```python
from build123d import *

# Parameters (mm, degrees)
SKETCH_1_W               = 29
SKETCH_1_H               = 32.7
EXTRUDE_1_DEPTH          = 29
SKETCH_2_R               = 14.5
SKETCH_2_R_2             = 12.5
EXTRUDE_2_DEPTH          = 7
SKETCH_3_R               = 1.5
CUT_EXTRUDE_1_DEPTH      = 5
CUT_EXTRUDE_START        = -2.9
SKETCH_4_R               = 1.5
CUT_EXTRUDE_2_DEPTH      = 2.9
SKETCH_5_R               = 4.3
SKETCH_5_R_2             = 3.5
EXTRUDE_3_DEPTH          = 6.9
SKETCH_6_W               = 16.3
SKETCH_6_H               = 15.8
EXTRUDE_4_DEPTH          = 2
PATTERN_CIRCULAR_1_COUNT = 4


with BuildPart() as part:
    # 草图1 → 凸台-拉伸1 (new body)
    with BuildSketch(Plane(origin=(0, 0, 0), x_dir=(1, 0, 0), z_dir=(0, 1, 0))):
        Rectangle(SKETCH_1_W, SKETCH_1_H)
    extrude(amount=EXTRUDE_1_DEPTH)

    # 草图2 → 凸台-拉伸2 (add)
    with BuildSketch(Plane.XY.offset(16.35)):
        with Locations((0, 14.5)):
            Circle(SKETCH_2_R)
        with Locations((0, 14.5)):
            Circle(SKETCH_2_R_2, mode=Mode.SUBTRACT)
    extrude(amount=EXTRUDE_2_DEPTH)

    # 草图3 → 切除-拉伸1 (cut)
    with BuildSketch(Plane.XZ):
        with Locations(Location((-10, 14.35, 0), (0, 0, 270))):
            Circle(SKETCH_3_R)
        with Locations(Location((10, 14.35, 0), (0, 0, 270))):
            Circle(SKETCH_3_R)
        with Locations(Location((-10, -14.35, 0), (0, 0, 270))):
            Circle(SKETCH_3_R)
        with Locations(Location((10, -14.35, 0), (0, 0, 270))):
            Circle(SKETCH_3_R)
    extrude(amount=-CUT_EXTRUDE_1_DEPTH, mode=Mode.SUBTRACT)

    # 草图4 → 切除-拉伸2 (cut)
    with BuildSketch(Plane(origin=(0, 29, 0), x_dir=(1, 0, 0), z_dir=(0, 1, 0)).offset(CUT_EXTRUDE_START)):
        with Locations(Location((0, 14.35, 0), (0, 0, 270))):
            Circle(SKETCH_4_R)
        with Locations(Location((-10, -14.35, 0), (0, 0, 90))):
            Circle(SKETCH_4_R)
        with Locations(Location((10, -14.35, 0), (0, 0, 90))):
            Circle(SKETCH_4_R)
    cut_extrude_2 = extrude(amount=CUT_EXTRUDE_2_DEPTH, mode=Mode.SUBTRACT)

    # 草图5 → 凸台-拉伸3 (add)
    with BuildSketch(Plane(origin=(0, 0, -16.35), x_dir=(-1, 0, 0), z_dir=(0, 0, -1))):
        with Locations(Location((-7.3, 21.8, 0), (0, 0, 180))):
            Circle(SKETCH_5_R)
        with Locations(Location((-7.3, 21.8, 0), (0, 0, 180))):
            Circle(SKETCH_5_R_2, mode=Mode.SUBTRACT)
    extrude(amount=EXTRUDE_3_DEPTH)

    # 草图6 → 凸台-拉伸4 (add)
    with BuildSketch(Plane(origin=(0, 0, -16.35), x_dir=(-1, 0, 0), z_dir=(0, 0, -1))):
        with Locations((0, 7.9)):
            Rectangle(SKETCH_6_W, SKETCH_6_H)
    extrude(amount=EXTRUDE_4_DEPTH)

    # 阵列(圆周)1: 切除-拉伸2 ×4 about axis, 1 skipped
    pattern_circular_1_axis = Axis((0, 14.5, 0), (0, 0, -1))
    add([cut_extrude_2.rotate(pattern_circular_1_axis, i * 360 / PATTERN_CIRCULAR_1_COUNT) for i in range(1, PATTERN_CIRCULAR_1_COUNT) if i not in (2,)], mode=Mode.SUBTRACT)


solid = part.part
```
Source: CAD feature listing. Evaluate the final solid. Frame: model axes, mm. A direction names the side the tool comes from. Round coordinates to 2 decimals unless told otherwise and drop trailing zeros. Loops run counter-clockwise (first coordinate to the right, second up) from the corner with the lowest first, then second, coordinate; pieces in that order, holes last. Notation, with made-up numbers: (-7.75, -36.75) - (17.25, -36.75) arc R20 cw to (17.25, -21.75) - close; hole circle Ø6 at (11, -24.5). An arc over 180 degrees is marked (long way). Use CSV: the item, a comma, the result in double quotes.
Q1. Section query D-D, the plane x = -3. Output: boundary loops of the cut face in (y, z).
Reported:
outline,"(0, -18.35) - (15.8, -18.35) - (15.8, -16.35) - (29, -16.35) - (29, 16.35) - (28.69, 16.35) - (28.69, 23.35) - (26.63, 23.35) - (26.63, 16.35) - (2.37, 16.35) - (2.37, 23.35) - (0.31, 23.35) - (0.31, 16.35) - (0, 16.35) - close"
Q2. Section query C-C, the plane z = -14.35. Output: boundary loops of the cut face in (x, y).
Reported:
outline,"(-14.5, 0) - (-11.5, 0) - (-11.5, 5) - (-8.5, 5) - (-8.5, 0) - (8.5, 0) - (8.5, 5) - (11.5, 5) - (11.5, 0) - (14.5, 0) - (14.5, 13) - (11.6, 13) - (11.6, 16) - (14.5, 16) - (14.5, 29) - (1.5, 29) - (1.5, 26.1) - (-1.5, 26.1) - (-1.5, 29) - (-14.5, 29) - (-14.5, 16) - (-11.6, 16) - (-11.6, 13) - (-14.5, 13) - close"
Q3. Section query B-B, the plane z = 20. Output: boundary loops of the cut face in (x, y).
Reported:
outline,"circle Ø29 at (0, 14.5); hole circle Ø25 at (0, 14.5)"
Q4. Pin query (flat end, axial travel): pin 1 Ø2 at (x, y) = (-4.5, 23.5) entering from -Z; pin 2 Ø6 at (x, y) = (1.5, 8) entering from -Z; pin 3 Ø7.5 at (x, y) = (6, 18) entering from +Z. Return the tip coordinate at first contact, or that it passes through.
Reported:
pin 1,"z = -16.35"
pin 2,"z = -18.35"
pin 3,"z = 16.35"
Q5. Reachability of faces 4 (the cylindrical face through (-10.07, 27.53, 15.85)), 5 (the cylindrical face through (13.03, 4.57, 15.85)), 6 (the cylindrical face through (-10.91, 2.46, -13.16)), 7 (the cylindrical face through (-13.03, 4.43, 15.85)), 8 (the cylindrical face through (5.77, 3.41, 19.8)) from +Z, -Z, +X, -X, +Y, -Y: full face, straight path, thin tool, end or side. Return the list, or none.
Reported:
face 4,"+Y"
face 5,"+X"
face 6,"-Y"
face 7,"-X"
face 8,"+Z"
Q6. Section query A-A, the plane y = 4.5. Output: boundary loops of the cut face in (x, z).
Reported:
outline,"(-14.5, -16.35) - (-8.15, -16.35) - (-8.15, -18.35) - (8.15, -18.35) - (8.15, -16.35) - (14.5, -16.35) - (14.5, 12.85) - (11.6, 12.85) - (11.6, 15.85) - (14.5, 15.85) - (14.5, 16.35) - (10.5, 16.35) - (10.5, 23.35) - (7.5, 23.35) - (7.5, 16.35) - (-7.5, 16.35) - (-7.5, 23.35) - (-10.5, 23.35) - (-10.5, 16.35) - (-14.5, 16.35) - (-14.5, 15.85) - (-11.6, 15.85) - (-11.6, 12.85) - (-14.5, 12.85) - close; hole circle Ø3 at (-10, -14.35); hole circle Ø3 at (-10, 14.35); hole circle Ø3 at (10, -14.35); hole circle Ø3 at (10, 14.35)"
Q7. Mould query, pull axis Z, two halves, no side actions, for faces 1 (the cylindrical face through (8.915, 24.905, -19.752)), 2 (the flat face through (-12, 25, 16.35)), 3 (the cylindrical face through (10.07, 2.46, -12.85)). Classes: pulls with the +Z half, pulls with the -Z half, needs draft (parallel to the pull), parting line crosses it, or undercut.
Reported:
face 1,"needs draft"
face 2,"pulls with the +Z half"
face 3,"undercut"
Q8. Ray query, line 1 along X through (y, z) = (27.35, 14.35); line 2 along Z through (x, y) = (-10, 27.45); line 3 along Z through (x, y) = (-11, 2.75). Return the intervals inside material, ascending.
Reported:
line 1,"-14.5 to -11.5, -8.5 to 8.5, 11.5 to 14.5"
line 2,"-16.35 to 12.85, 15.85 to 16.35"
line 3,"-16.35 to -15.47, -13.23 to 13.23, 15.47 to 16.35"
